Autodesk Fusion 360 part; units mm, degrees
sketch "Sketch1" plane through (0, 0, 0) normal (0, 0, 1) x (1, 0, 0)
  circle A0 centre (0, 0) radius 10
  dimension "d1" = 20
extrude "Extrude1" add sketch "Sketch1" along normal blind 2
sketch "Sketch2" plane through (0, 0, 2) normal (0, 0, 1) x (-1, 0, 0)
  circle A0 centre (0, 0) radius 10
  circle A1 centre (0, 0) radius 8.5
  dimension "d4" = 17
extrude "Extrude2" add sketch "Sketch2" along normal blind 30 contours A1
sketch "Sketch3" plane through (0, 0, 32) normal (0, 0, 1) x (-1, 0, 0)
  circle A0 centre (0, 0) radius 8.5
  circle A1 centre (0, 0) radius 6.1
  dimension "d7" = 12.2
extrude "Extrude3" cut sketch "Sketch3" against normal blind 60 contours A1
chamfer "Chamfer1" distance 0.5 distance2 1 2 edges at (5.6872, 2.2059, 0) (7.9248, 3.0737, 32) measured on face at (8.6401, -0.7999, 0) measured on face at (-7.6684, 0.4223, 32)
Source: CAD feature listing. Evaluate the final solid. Frame: model axes, mm. A direction names the side the tool comes from. Round coordinates to 2 decimals unless told otherwise and drop trailing zeros. Loops run counter-clockwise (first coordinate to the right, second up) from the corner with the lowest first, then second, coordinate; pieces in that order, holes last. Notation, with made-up numbers: M -19.75,-13 L 28.25,-13 A21 ccw 28.25,-1 Z; hole C 15.5,45.25 d4. An arc over 180 degrees is marked long. Answer as CSV lines item,"result".
Q1. Cut plane C-C (z = 16.5). Return the cut outline in (x, y), plus the area to 3 significant figures.
Verdict:
outline,"C 0,0 d17; hole C 0,0 d12.2"
area,"110 mm^2"
Q2. Cut plane A-A (y = 0). Return the cut outline in (x, z), plus the area to 3 significant figures.
Verdict:
outline,"M -10,0 L -6.6,0 L -6.1,1 L -6.1,32 L -8,32 L -8.5,31 L -8.5,2 L -10,2 Z; M 6.1,1 L 6.6,0 L 10,0 L 10,2 L 8.5,2 L 8.5,31 L 8,32 L 6.1,32 Z"
area,"159 mm^2"
Q3. Contact query for flat-ended pins moving along their axis: pin 1 (1.5 mm diameter, centred on y = 4, z = 25.5, fed in from +X); pin 2 (4 mm diameter, centred on x = -5.5, z = 6.5, fed in from +Y); pin 3 (10 mm diameter, centred on x = -5.5, z = 27, fed in from -Y). Output: stop coordinate, or through.
Verdict:
pin 1,"stops at x = 7.85"
pin 2,"stops at y = 7.75"
pin 3,"stops at y = -8.49"
Q4. Pull-direction query (X, two-part tool) for faces 1 (the face through (2, 6, 32)), 2 (the face through (6.094, -0.268, 16.717)), 3 (the face through (-2.17, 9.76, 0.99)); classes: +X half, -X half, draft (parallel to the pull), parting line (faces both ways), or undercut.
Verdict:
face 1,"draft"
face 2,"undercut"
face 3,"parting line"
Q5. Reachability of faces 4 (the face through (7, -2, 0)), 5 (the face through (-4.5, -7.4, 2)) from +Z, -Z, +X, -X, +Y, -Y: full face, straight path, thin tool, end or side. Return the list, or none.
Verdict:
face 4,"-Z, +X, -X, +Y, -Y"
face 5,"+Z"
Q6. Line query: line 1 along Y through (x, z) = (0, 18.5); line 2 along Z through (x, y) = (7.5, 5). Output: solid intervals per line, ascending.
Verdict:
line 1,"y = -8.5 to -6.1, 6.1 to 8.5"
line 2,"z = 0 to 2"
